```python
from build123d import *

# Parameters (mm, degrees)
F0_W     = 3
F0_H     = 13
F1_DEPTH = 8
F2_R     = 3
F3_DEPTH = 10
F4_DEPTH = 25
F5_DEPTH = 15
F6_R     = 1.75
F7_DEPTH = 25


with BuildPart() as f1:
    # F0 (on Top) → F1 (new body)
    with BuildSketch(Plane.XY):
        with Locations((-36.0112562776, 16.7272449248)):
            Rectangle(F0_W, F0_H)
        with Locations((-30.0112562776, 16.7272449248)):
            Rectangle(F0_W, F0_H)
        Polygon((-34.5112562776, 10.2272449248), (-37.5112562776, 10.2272449248), (-37.5112562776, 5.2272449248), (-28.5112562776, 5.2272449248), (-28.5112562776, 10.2272449248), (-31.5112562776, 10.2272449248), align=None)
    extrude(amount=F1_DEPTH)

    # F2 (on face) → F3 (cut)
    with BuildSketch(Plane.YZ.offset(-28.5112562776)):
        with Locations((17.2272449248, 4)):
            Circle(F2_R)
    extrude(amount=-F3_DEPTH, mode=Mode.SUBTRACT)

    # F2 (on face) → F4 (cut)
    with BuildSketch(Plane.YZ.offset(-28.5112562776)):
        with BuildLine():
            ThreePointArc((20.2339589596, 8), (23.1952457023, 3.989991066), (20.2070418745, 0))
            Line((20.2070418745, 0), (23.2272449248, 0))
            Line((23.2272449248, 0), (23.2272449248, 8))
            Line((23.2272449248, 8), (20.2339589596, 8))
        make_face()
    extrude(amount=-F4_DEPTH, mode=Mode.SUBTRACT)

    # F5 (add): a face of the model
    f5_faces = [f1.faces().sort_by_distance(p)[0] for p in [
        (-33.0112562776, 5.2272449248, 4),
    ]]
    extrude(f5_faces, amount=F5_DEPTH)

    # F6 (on face) → F7 (cut)
    with BuildSketch(Plane.YZ.offset(-28.5112562776)):
        with Locations((-5.0227550752, 3.25)):
            Circle(F6_R)
    extrude(amount=-F7_DEPTH, mode=Mode.SUBTRACT)


solid = f1.part
```
Design review of the part built by this model. Coordinates are the model's own, in mm. A direction names the side the tool comes from. Give positions to 0.01 mm unless a question says otherwise; leave off trailing zeros. Write each loop counter-clockwise with the first axis right and the second up, starting at its lowest first coordinate (ties: lowest second). Pieces come first, ordered by that corner, then holes.
(1) Clearance check with flat-ended pins moving along their axes: pin 1 Ø1.5 at (x, z) = (-32.5, 5.5) entering from +Y; pin 2 Ø1 at (x, y) = (-34.5, -1.5) entering from -Z. State where each tip first meets the part, or that it passes through.
Checked values:
pin 1: stops at y = 10.23
pin 2: stops at z = 0
(2) Add section C-C (z = 4). Give the boundary of the cut face in (x, y).
Checked values:
outline: (-37.51, -9.77) - (-28.51, -9.77) - (-28.51, -6.6) - (-37.51, -6.6) - close; (-37.51, -3.44) - (-28.51, -3.44) - (-28.51, 14.23) - (-31.51, 14.23) - (-31.51, 10.23) - (-34.51, 10.23) - (-34.51, 14.23) - (-37.51, 14.23) - close; (-37.51, 20.23) - (-34.51, 20.23) - (-34.51, 23.2) - (-37.51, 23.2) - close; (-31.51, 20.23) - (-28.51, 20.23) - (-28.51, 23.2) - (-31.51, 23.2) - close
(3) Add section B-B (x = -37). Give the boundary of the cut face in (y, z).
Checked values:
outline: (-9.77, 0) - (20.21, 0) arc R4.18 ccw to (20.23, 8) - (-9.77, 8) - close; hole circle Ø3.5 at (-5.02, 3.25); hole circle Ø6 at (17.23, 4)
(4) Mouldability with a two-part tool opening along Z and no side actions: class faces 3 (the face through (-28.511, 7, 4)), 4 (the face through (-32.948, -6.411, 2.185)), 5 (the face through (-33, 5, 8)), 6 (the face through (-35.99, 23.195, 4.065)) as +Z half, -Z half, draft (parallel to the pull), parting line (faces both ways), or undercut.
Checked values:
face 3: draft
face 4: undercut
face 5: +Z half
face 6: parting line
(5) Wall thickness on line 1 along X through (y, z) = (21.5, 7.25); line 2 along Y through (x, z) = (-28.75, 3); line 3 along Y through (x, z) = (-34.75, 4.75): over which ranges is each line inside the solid? List them lowest first.
Checked values:
line 1: x = -37.51 to -34.51, -31.51 to -28.51
line 2: y = -9.77 to -6.75, -3.29 to 14.4, 20.06 to 23.07
line 3: y = -9.77 to -5.92, -4.12 to 14.32, 20.13 to 23.13
(6) Add section A-A (y = 11.5). Give the boundary of the cut face in (x, z).
Checked values:
outline: (-37.51, 0) - (-34.51, 0) - (-34.51, 8) - (-37.51, 8) - close; (-31.51, 0) - (-28.51, 0) - (-28.51, 8) - (-31.51, 8) - close
(7) Tool access review of faces 1 (the face through (-35.99, 20, 2.85)), 2 (the face through (-34.511, 14, 4)): name each direction out of +Z, -Z, +X, -X, +Y, -Y from which nothing blocks a thin tool from reaching the whole face with its end or side.
Checked values:
face 1: +X, -X
face 2: +Z, -Z, +Y
(8) Add section D-D (x = -33.5). Give the boundary of the cut face in (y, z).
Checked values:
outline: (-9.77, 0) - (10.23, 0) - (10.23, 8) - (-9.77, 8) - close; hole circle Ø3.5 at (-5.02, 3.25)
